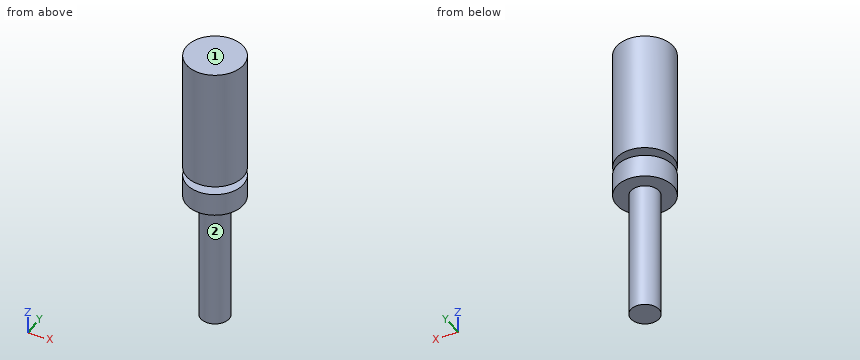
```python
from build123d import *

# Parameters (mm, degrees)
F0_R     = 3.175
F2_DEPTH = 31.75
F1_R     = 6.35
F3_DEPTH = 2.54
F5_R     = 6.35
F6_DEPTH = 27.49417


with BuildPart() as f2:
    # F0 (on Top) → F2 (new body, symmetric)
    with BuildSketch(Plane.XY):
        Circle(F0_R)
    extrude(amount=F2_DEPTH, both=True)

    # F1 (on Top) → F3 (join, symmetric)
    with BuildSketch(Plane.XY):
        Circle(F1_R)
    extrude(amount=F3_DEPTH, both=True)

    # F5 (on offset) → F6 (join)
    with BuildSketch(Plane.XY.offset(4.445)):
        Circle(F5_R)
    extrude(amount=F6_DEPTH)


solid = f2.part
```
Can you work these out from the model? Positions are in its coordinate system, mm. Face numbers are marked on the shaded views. A direction names the side the tool comes from. Round coordinates to 2 decimals unless told otherwise and drop trailing zeros. Loops run counter-clockwise (first coordinate to the right, second up) from the corner with the lowest first, then second, coordinate; pieces in that order, holes last. Notation, with made-up numbers: (55.25, -37) -> (77.25, -37) arc R16 ccw to (77.25, -29) -> close; hole circle Ø4 at (7, 36.25). An arc over 180 degrees is marked (long way). One line per item, written item: value. Start each with the question number.
1. If we section it at C-C, the plane y = -5.5: Write out the boundary of the cut face in (x, z) (3 decimals).
2. If I drill on probe 1 along Z at (x, y) = (-5, -1.75) (3 decimals); probe 2 along X at (y, z) = (0.25, 21.5); probe 3 along Y at (x, z) = (5.5, 14.5), over which ranges is the centre line in solid material (lowest first)?
3. For the marked faces 1 and 2, which set-ups out of +Z, -Z, +X, -X, +Y, -Y let a thin tool reach every point of the face, with its end or its side?
4. If we section it at A-A, the plane y = 0: Write out the boundary of the cut face in (x, z) (3 decimals), then the cut area to 3 significant figures.
5. If we section it at D-D, the plane z = 6.5: Write out the boundary of the cut face in (x, y), then the cut area to 3 significant figures.
6. For pin 1 (4 mm diameter, centred on x = 5, y = -2, fed in from -Z); pin 2 (2 mm diameter, centred on x = -1.5, z = -2, fed in from -Y), each with a flat end and sliding along its axis, tell me the tip position at first contact or that it passes through.
Calculated:
1. outline: (-3.174, -2.54) -> (3.174, -2.54) -> (3.174, 2.54) -> (-3.174, 2.54) -> close; (-3.174, 4.445) -> (3.174, 4.445) -> (3.174, 31.939) -> (-3.174, 31.939) -> close
2. probe 1: z = -2.54 to 2.54, 4.445 to 31.939
2. probe 2: x = -6.35 to 6.35
2. probe 3: y = -3.17 to 3.17
3. face 1: +Z, +X, -X, +Y, -Y
3. face 2: -Z
4. outline: (-6.35, -2.54) -> (-3.175, -2.54) -> (-3.175, -31.75) -> (3.175, -31.75) -> (3.175, -2.54) -> (6.35, -2.54) -> (6.35, 2.54) -> (3.175, 2.54) -> (3.175, 4.445) -> (6.35, 4.445) -> (6.35, 31.939) -> (-6.35, 31.939) -> (-6.35, 4.445) -> (-3.175, 4.445) -> (-3.175, 2.54) -> (-6.35, 2.54) -> close
4. area: 611 mm²
5. outline: circle Ø12.7 at (0, 0)
5. area: 127 mm²
6. pin 1: stops at z = -2.54
6. pin 2: stops at y = -6.33
